Read the model definition and answer for the solid it produces. Units are mm, in the model's axes. Face numbers are marked on the shaded views. A direction names the side the tool comes from. Coordinates: 2 decimals unless noted, no trailing zeros. Write each loop counter-clockwise with the first axis right and the second up, starting at its lowest first coordinate (ties: lowest second). Pieces come first, ordered by that corner, then holes. Notation, with made-up numbers: (-5.5, 51) -> (29.5, 51) arc R20 cw to (29.5, 86) -> close; hole circle Ø9 at (57.25, 68). An arc over 180 degrees is marked (long way). Use CSV: the item, a comma, the result in double quotes.
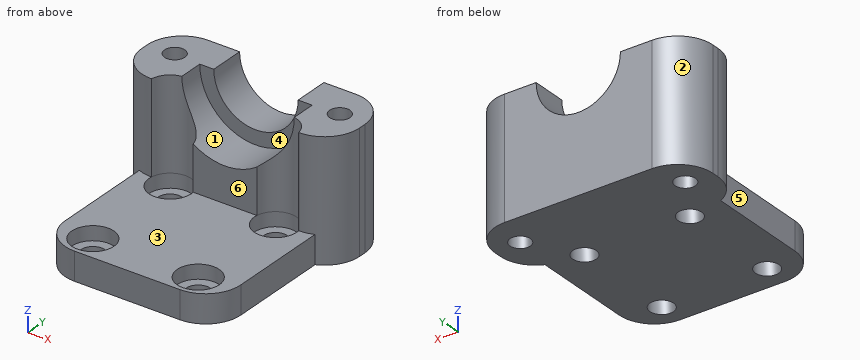
from build123d import *

# Parameters (mm, degrees)
F0_W      = 25
F0_H      = 30
F1_DEPTH  = 4
F2_R      = 1.675
F3_DEPTH  = 25
F4_W      = 25
F4_H      = 11
F5_DEPTH  = 13
F7_DEPTH  = 6
F8_R      = 8
F9_DEPTH  = 6
F2_R_2    = 3
F10_DEPTH = 2
F11_W     = 11
F11_H     = 17
F12_DEPTH = 3
F13_R     = 5
F14_W     = 11
F14_H     = 17
F15_DEPTH = 3
F16_R     = 1.45
F17_DEPTH = 25
F18_R     = 5
F19_DEPTH = 25


with BuildPart() as f1:
    # F0 (on Top) → F1 (new body)
    with BuildSketch(Plane.XY):
        with Locations((12.5, 15)):
            Rectangle(F0_W, F0_H)
    extrude(amount=F1_DEPTH)

    # F2 (on face) → F3 (cut)
    with BuildSketch(Plane.XY.offset(4)):
        with BuildLine():
            ThreePointArc((3.325, 18.5605346784), (5, 16.8855346784), (6.675, 18.5605346784))
            ThreePointArc((6.675, 18.5605346784), (5, 20.2355346784), (3.325, 18.5605346784))
        make_face()
        with Locations((20, 18.5605346784)):
            Circle(F2_R)
        with Locations((20, 3.5605346784)):
            Circle(F2_R)
        with Locations((5, 3.5605346784)):
            Circle(F2_R)
    extrude(amount=-F3_DEPTH, mode=Mode.SUBTRACT)

    # F4 (on face) → F5 (join)
    with BuildSketch(Plane.XY.offset(4)):
        with Locations((12.5, 24.5)):
            Rectangle(F4_W, F4_H)
    extrude(amount=F5_DEPTH)

    # F6 (on face) → F7 (cut)
    with BuildSketch(Plane(origin=(0, 30, 0), x_dir=(-1, 0, 0), z_dir=(0, 1, 0))):
        with BuildLine():
            ThreePointArc((-18.5, 17), (-12.5, 11), (-6.5, 17))
            Line((-6.5, 17), (-18.5, 17))
        make_face()
    extrude(amount=-F7_DEPTH, mode=Mode.SUBTRACT)

    # F8 (on face) → F9 (cut)
    with BuildSketch(Plane.XZ.offset(-19)):
        with Locations((12.5, 17)):
            Circle(F8_R)
    extrude(amount=-F9_DEPTH, mode=Mode.SUBTRACT)

    # F2 (on face) → F10 (cut)
    with BuildSketch(Plane.XY.offset(4)):
        with BuildLine():
            ThreePointArc((8, 18.5605346784), (5, 21.5605346784), (2, 18.5605346784))
            ThreePointArc((2, 18.5605346784), (5, 15.5605346784), (8, 18.5605346784))
        make_face()
        with BuildLine():
            ThreePointArc((3.325, 18.5605346784), (5, 20.2355346784), (6.675, 18.5605346784))
            ThreePointArc((6.675, 18.5605346784), (5, 16.8855346784), (3.325, 18.5605346784))
        make_face(mode=Mode.SUBTRACT)
        with Locations((20, 18.5605346784)):
            Circle(F2_R_2)
        with Locations((20, 18.5605346784)):
            Circle(F2_R, mode=Mode.SUBTRACT)
        with Locations((20, 3.5605346784)):
            Circle(F2_R_2)
        with Locations((20, 3.5605346784)):
            Circle(F2_R, mode=Mode.SUBTRACT)
        with Locations((5, 3.5605346784)):
            Circle(F2_R_2)
        with Locations((5, 3.5605346784)):
            Circle(F2_R, mode=Mode.SUBTRACT)
    extrude(amount=-F10_DEPTH, mode=Mode.SUBTRACT)

    # F11 (on face) → F12 (join)
    with BuildSketch(Plane(origin=(0, 0, 0), x_dir=(0, -1, 0), z_dir=(-1, 0, 0))):
        with Locations((-24.5, 8.5)):
            Rectangle(F11_W, F11_H)
    extrude(amount=F12_DEPTH)

    # F13
    f13_edges = [f1.edges().sort_by_distance(p)[0] for p in [
        (0, 0, 2),
        (25, 0, 2),
    ]]
    fillet(f13_edges, radius=F13_R)

    # F14 (on face) → F15 (join)
    with BuildSketch(Plane.YZ.offset(25)):
        with Locations((24.5, 8.5)):
            Rectangle(F14_W, F14_H)
    extrude(amount=F15_DEPTH)

    # F16 (on face) → F17 (cut)
    with BuildSketch(Plane.XY.offset(17)):
        with Locations((0.7500000062, 25.25)):
            Circle(F16_R)
        with Locations((24.2500000062, 25.25)):
            Circle(F16_R)
    extrude(amount=-F17_DEPTH, mode=Mode.SUBTRACT)

    # F18
    f18_edges = [f1.edges().sort_by_distance(p)[0] for p in [
        (-3, 19, 8.5),
        (28, 19, 8.5),
        (28, 30, 8.5),
        (-3, 30, 8.5),
    ]]
    fillet(f18_edges, radius=F18_R)

    # F2 (on face) → F19 (cut)
    with BuildSketch(Plane.XY.offset(4)):
        with BuildLine():
            ThreePointArc((8, 18.5605346784), (5, 21.5605346784), (2, 18.5605346784))
            ThreePointArc((2, 18.5605346784), (5, 15.5605346784), (8, 18.5605346784))
        make_face()
        with BuildLine():
            ThreePointArc((3.325, 18.5605346784), (5, 20.2355346784), (6.675, 18.5605346784))
            ThreePointArc((6.675, 18.5605346784), (5, 16.8855346784), (3.325, 18.5605346784))
        make_face(mode=Mode.SUBTRACT)
        with Locations((20, 18.5605346784)):
            Circle(F2_R_2)
        with Locations((20, 18.5605346784)):
            Circle(F2_R, mode=Mode.SUBTRACT)
        with BuildLine():
            ThreePointArc((3.325, 18.5605346784), (5, 16.8855346784), (6.675, 18.5605346784))
            ThreePointArc((6.675, 18.5605346784), (5, 20.2355346784), (3.325, 18.5605346784))
        make_face()
        with Locations((20, 18.5605346784)):
            Circle(F2_R)
    extrude(amount=F19_DEPTH, mode=Mode.SUBTRACT)


solid = f1.part
1. Each of these flat-tipped pins is pushed along its axis until it touches: pin 1 Ø9.5 at (x, y) = (5, 18.56) entering from +Z; pin 2 Ø2 at (x, y) = (20, 18.56) entering from -Z; pin 3 Ø1.8 at (x, y) = (6.5, 18.5) entering from +Z; pin 4 Ø6 at (y, z) = (5, 4) entering from -X. Where does it stop, or does it pass through?
Solutions:
pin 1,"stops at z = 17"
pin 2,"passes through"
pin 3,"stops at z = 2"
pin 4,"stops at x = 0"
2. A cutting plane is placed at B-B (x = 12.5). Give the vertices of the cut face in (y, z).
Solutions:
outline,"(0, 0) -> (30, 0) -> (30, 11) -> (25, 11) -> (25, 9) -> (19, 9) -> (19, 4) -> (0, 4) -> close"
3. A tool of negligible diameter and unlimited length cuts with its end or side. For the marked faces 4, 5 and 6, from which of +Z, -Z, +X, -X, +Y, -Y can it reach the whole face along a straight path? Write none if from no direction.
Solutions:
face 4,"+Z, -Y"
face 5,"+Z, -Z, -X, -Y"
face 6,"+Z, +X, -X, -Y"
4. A cutting plane is placed at D-D (x = 24.25). Give the vertices of the cut face in (y, z), and give its area (3 significant figures).
Solutions:
outline,"(2.37, 0) -> (23.8, 0) -> (23.8, 17) -> (19.16, 17) -> (19.16, 4) -> (2.37, 4) -> close; (26.7, 0) -> (29.84, 0) -> (29.84, 17) -> (26.7, 17) -> close"
area,"199 mm^2"
5. For a pull along X with two mould halves and no side action, classify the marked faces 1, 2 and 3 as pulls with the +X half, pulls with the -X half, needs draft (parallel to the pull), parting line crosses it, or undercut.
Solutions:
face 1,"undercut"
face 2,"pulls with the -X half"
face 3,"needs draft"
6. Find the intervals of material crossed by line 1 along Y through (x, z) = (5, 2.85); line 2 along Y through (x, z) = (20, 0.75); line 3 along X through (y, z) = (18.5, 2.25), in increasing order.
Solutions:
line 1,"y = 0 to 0.56, 6.56 to 15.56, 21.56 to 30"
line 2,"y = 0 to 1.89, 5.24 to 16.89, 20.24 to 30"
line 3,"x = 0 to 2, 8 to 17, 23 to 25"
7. A cutting plane is placed at A-A (z = 11.5). Give the number of separate pieces and of enclosed holes in the cut face, and give its area (3 significant figures).
Solutions:
separate pieces,"2"
enclosed holes,"2"
area,"193 mm^2"
